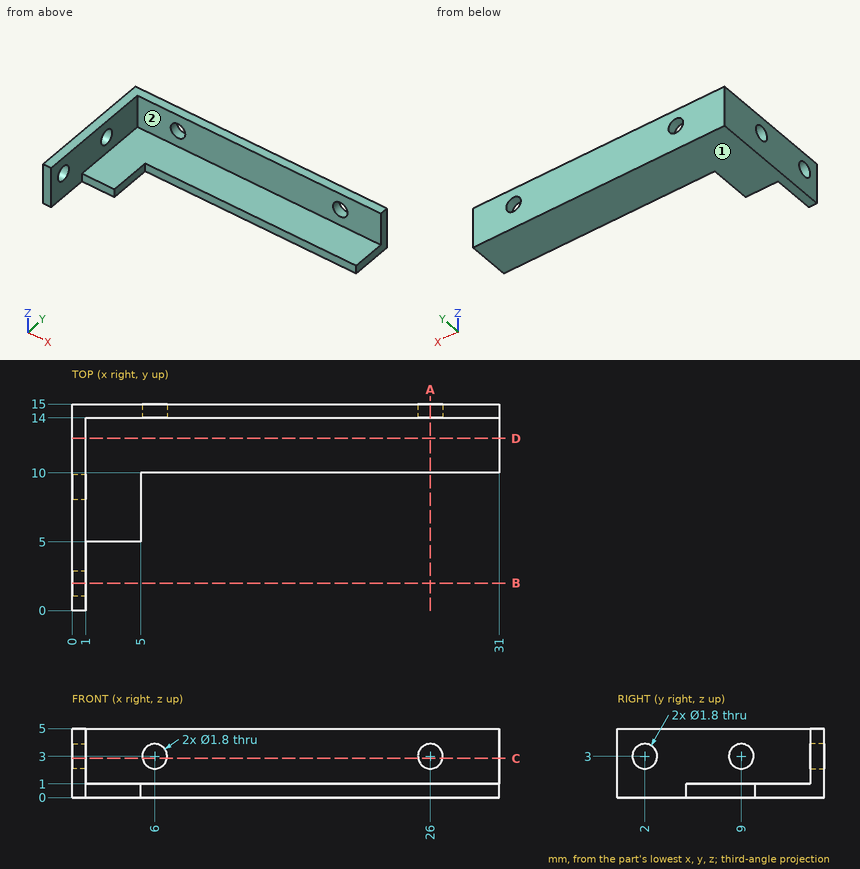
Geometry check sheet. Reference: drawing and pictorial views, mm from the part's lowest x, y, z. A direction names the side the tool comes from. Coordinates: 2 decimals unless noted, no trailing zeros. Write each loop counter-clockwise with the first axis right and the second up, starting at its lowest first coordinate (ties: lowest second). Pieces come first, ordered by that corner, then holes. Notation, with made-up numbers: M 11,11.5 L 62,11.5 A21 cw 62,24.5 Z; hole C 22,18 d3. An arc over 180 degrees is marked long. Write item = value, one per line. Start each with the question number.
1. Sectioned sample at C-C (z = 2.85). Record the cut outline in (x, y).
2. Sectioned sample at D-D (y = 12.5). Record the cut outline in (x, z), then the cut area to 3 significant figures.
3. Go/stop test with flat-tipped pins: pin 1 (1.2 mm diameter, centred on x = 9, z = 4, fed in from -Y); pin 2 (1.1 mm diameter, centred on x = 16, z = 0.5, fed in from -Y); pin 3 (1.5 mm diameter, centred on y = 2, z = 3.5, fed in from +X). Record where each tip stops, or that it passes through.
4. Sectioned sample at B-B (y = 2). Record the cut outline in (x, z), then the cut area to 3 significant figures.
5. Sectioned sample at A-A (x = 26). Record the cut outline in (y, z).
6. Thickness scan on probe 1 along X at (y, z) = (14.8, 3); probe 2 along Y at (x, z) = (0.5, 3); probe 3 along Y at (x, z) = (11.5, 2.6). Record the ranges inside material, lowest first.
7. Tool access check on the marked faces 1 and 2. Record the directions out of +Z, -Z, +X, -X, +Y, -Y that give a thin tool (end or side, any length) a straight path to the whole face; none if there is none.
The answers:
q1.outline = M 0,0 L 1,0 L 1,1.11 L 0,1.11 Z; M 0,2.89 L 1,2.89 L 1,8.11 L 0,8.11 Z; M 0,9.89 L 1,9.89 L 1,14 L 5.11,14 L 5.11,15 L 0,15 Z; M 6.89,14 L 25.11,14 L 25.11,15 L 6.89,15 Z; M 26.89,14 L 31,14 L 31,15 L 26.89,15 Z
q2.outline = M 0,0 L 31,0 L 31,1 L 1,1 L 1,5 L 0,5 Z
q2.area = 35.0 mm²
q3.pin_1 = 14
q3.pin_2 = 10
q3.pin_3 = 1
q4.outline = M 0,0 L 1,0 L 1,2.1 L 0,2.1 Z; M 0,3.9 L 1,3.9 L 1,5 L 0,5 Z
q4.area = 3.20 mm²
q5.outline = M 10,0 L 15,0 L 15,2.1 L 14,2.1 L 14,1 L 10,1 Z; M 14,3.9 L 15,3.9 L 15,5 L 14,5 Z
q6.probe_1 = 0 to 5.1, 6.9 to 25.1, 26.9 to 31
q6.probe_2 = 0 to 1.1, 2.9 to 8.1, 9.9 to 15
q6.probe_3 = 14 to 15
q7.face_1 = -Z, +X, -X, +Y, -Y
q7.face_2 = +Z, +X, -Y
